CAD build for the part. Positions are in the model's coordinates, mm. Face numbers are marked on the shaded views. A direction names the side the tool comes from. Round coordinates to 2 decimals unless told otherwise and drop trailing zeros. Loops run counter-clockwise (first coordinate to the right, second up) from the corner with the lowest first, then second, coordinate; pieces in that order, holes last.
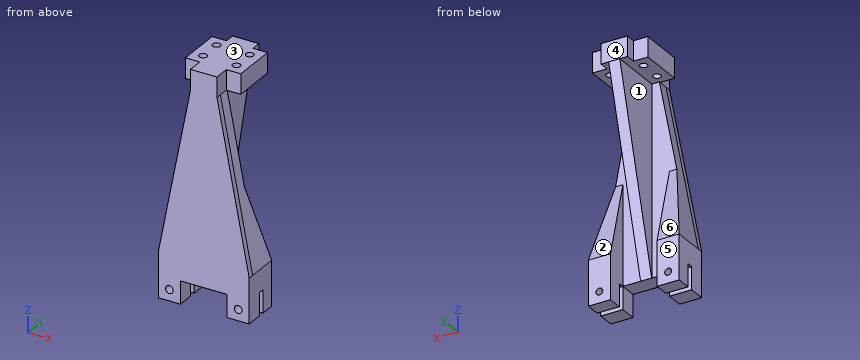
```python
from build123d import *

# Parameters (mm, degrees)
SKETCH1_W            = 41
SKETCH1_H            = 100.5
BOSS_EXTRUDE1_DEPTH  = 5
SKETCH2_W            = 21
SKETCH2_H            = 10.2
CUT_EXTRUDE1_DEPTH   = 109.656569061
SKETCH9_R            = 1.75
CUT_EXTRUDE4_DEPTH   = 109.656569061
CUT_EXTRUDE5_DEPTH   = 109.656569061
BOSS_EXTRUDE4_DEPTH  = 23.9
SKETCH16_W           = 5
SKETCH16_H           = 85.3
BOSS_EXTRUDE5_DEPTH  = 23.9
CUT_EXTRUDE8_DEPTH   = 108.072218619
BOSS_EXTRUDE6_DEPTH  = 28.9
SKETCH25_W           = 6.53486924
SKETCH25_H           = 4.45
CUT_EXTRUDE9_DEPTH   = 108.872424651
SKETCH26_R           = 1.75
CUT_EXTRUDE10_DEPTH  = 113.323016341
SKETCH27_R           = 1.75
BOSS_EXTRUDE7_DEPTH  = 2.5
BOSS_EXTRUDE8_START  = 4
SKETCH28_R           = 1.75
BOSS_EXTRUDE8_DEPTH  = 4
SKETCH29_W           = 10
SKETCH29_H           = 10
BOSS_EXTRUDE9_DEPTH  = 2.7
SKETCH30_W           = 10
SKETCH30_H           = 20.2
BOSS_EXTRUDE10_DEPTH = 6.6
SKETCH31_R           = 1.55
CUT_EXTRUDE11_DEPTH  = 6.6
CHAMFER2_SIZE        = 34.7
CHAMFER2_SIZE_2      = 9.297836977


with BuildPart() as part:
    # Sketch1 → Boss-Extrude1 (new body)
    with BuildSketch(Plane(origin=(0, 0, 0), x_dir=(1, 0, 0), z_dir=(0, 1, 0))):
        with Locations((20.5, 50.25)):
            Rectangle(SKETCH1_W, SKETCH1_H)
    extrude(amount=BOSS_EXTRUDE1_DEPTH)

    # Sketch2 → Cut-Extrude1 (cut, through all)
    with BuildSketch(Plane(origin=(0, 5, 0), x_dir=(1, 0, 0), z_dir=(0, 1, 0))):
        with Locations((20.5, 95.4)):
            Rectangle(SKETCH2_W, SKETCH2_H)
    extrude(amount=-CUT_EXTRUDE1_DEPTH, mode=Mode.SUBTRACT)

    # Sketch9 → Cut-Extrude4 (cut, through all)
    with BuildSketch(Plane(origin=(0, 5, 0), x_dir=(1, 0, 0), z_dir=(0, 1, 0))):
        with Locations(Location((5, 95.5, 0), (0, 0, 270))):
            Circle(SKETCH9_R)
        with Locations(Location((36, 95.5, 0), (0, 0, 270))):
            Circle(SKETCH9_R)
    extrude(amount=-CUT_EXTRUDE4_DEPTH, mode=Mode.SUBTRACT)

    # Sketch11 → Cut-Extrude5 (cut, through all)
    with BuildSketch(Plane(origin=(0, 5, 0), x_dir=(1, 0, 0), z_dir=(0, 1, 0))):
        Polygon((15.5, 0), (0, 80.3), (0, 0), align=None)
        Polygon((25.5, 0), (41, 80.3), (41, 0), align=None)
    extrude(amount=-CUT_EXTRUDE5_DEPTH, mode=Mode.SUBTRACT)

    # Sketch12 → Boss-Extrude4 (add)
    with BuildSketch(Plane(origin=(0, 5, 0), x_dir=(1, 0, 0), z_dir=(0, 1, 0))):
        Polygon((25.5, 0), (15.5, 0), (14.53486924, 5), (26.46513076, 5), align=None)
    extrude(amount=BOSS_EXTRUDE4_DEPTH)

    # Sketch16 → Boss-Extrude5 (add)
    with BuildSketch(Plane(origin=(0, 5, 0), x_dir=(1, 0, 0), z_dir=(0, 1, 0))):
        with Locations((20.5, 47.65)):
            Rectangle(SKETCH16_W, SKETCH16_H)
    extrude(amount=BOSS_EXTRUDE5_DEPTH)

    # Sketch17 → Cut-Extrude8 (cut, through all)
    with BuildSketch(Plane.ZY.offset(-18)):
        Polygon((-90.4, 5), (-5, 28.9), (-90.3, 28.9), align=None)
    extrude(amount=-CUT_EXTRUDE8_DEPTH, mode=Mode.SUBTRACT)

    # Sketch23 → Boss-Extrude6 (add)
    with BuildSketch(Plane(origin=(0, 28.9, 0), x_dir=(1, 0, 0), z_dir=(0, 1, 0))):
        Polygon((26.46513076, 5), (33, 5), (33, 0), (25.5, 0), align=None)
        Polygon((14.53486924, 5), (8, 5), (8, 0), (15.5, 0), align=None)
    extrude(amount=-BOSS_EXTRUDE6_DEPTH)

    # Sketch25 → Cut-Extrude9 (cut, through all)
    with BuildSketch(Plane(origin=(0, 0, -5), x_dir=(-1, 0, 0), z_dir=(0, 0, -1))):
        with Locations((-11.26743462, 2.225)):
            Rectangle(SKETCH25_W, SKETCH25_H)
        with Locations((-29.73256538, 2.225)):
            Rectangle(SKETCH25_W, SKETCH25_H)
        with Locations((-11.26743462, 26.675)):
            Rectangle(SKETCH25_W, SKETCH25_H)
        with Locations((-29.73256538, 26.675)):
            Rectangle(SKETCH25_W, SKETCH25_H)
    extrude(amount=-CUT_EXTRUDE9_DEPTH, mode=Mode.SUBTRACT)

    # Sketch26 → Cut-Extrude10 (cut, through all)
    with BuildSketch(Plane.XY):
        with Locations((13, 19.45)):
            Circle(SKETCH26_R)
        with Locations((28, 19.45)):
            Circle(SKETCH26_R)
        with Locations((13, 9.45)):
            Circle(SKETCH26_R)
        with Locations((28, 9.45)):
            Circle(SKETCH26_R)
    extrude(amount=-CUT_EXTRUDE10_DEPTH, mode=Mode.SUBTRACT)

    # Sketch27 → Boss-Extrude7 (add)
    with BuildSketch(Plane.XZ):
        Polygon((26.46513076, -5), (26.46513076, 0), (14.53486924, 0), (14.53486924, -5), (0, -80.3), (0, -100.5), (10, -100.5), (10, -90.3), (31, -90.3), (31, -100.5), (41, -100.5), (41, -80.3), align=None)
        with Locations(Location((5, -95.5, 0), (0, 0, 90))):
            Circle(SKETCH27_R, mode=Mode.SUBTRACT)
        with Locations(Location((36, -95.5, 0), (0, 0, 90))):
            Circle(SKETCH27_R, mode=Mode.SUBTRACT)
    extrude(amount=BOSS_EXTRUDE7_DEPTH)

    # Sketch28 → Boss-Extrude8 (add)
    with BuildSketch(Plane.XY.offset(BOSS_EXTRUDE8_START)):
        Polygon((26.46513076, -2.5), (26.46513076, 4.45), (33, 4.45), (33, 24.45), (26.46513076, 24.45), (26.46513076, 28.9), (14.53486924, 28.9), (14.53486924, 24.45), (8, 24.45), (8, 4.45), (14.53486924, 4.45), (14.53486924, -2.5), align=None)
        with Locations((28, 9.45)):
            Circle(SKETCH28_R, mode=Mode.SUBTRACT)
        with Locations((13, 9.45)):
            Circle(SKETCH28_R, mode=Mode.SUBTRACT)
        with Locations((28, 19.45)):
            Circle(SKETCH28_R, mode=Mode.SUBTRACT)
        with Locations((13, 19.45)):
            Circle(SKETCH28_R, mode=Mode.SUBTRACT)
    extrude(amount=-BOSS_EXTRUDE8_DEPTH)

    # Sketch29 → Boss-Extrude9 (add)
    with BuildSketch(Plane(origin=(0, 5, 0), x_dir=(1, 0, 0), z_dir=(0, 1, 0))):
        with Locations((36, 85.3)):
            Rectangle(SKETCH29_W, SKETCH29_H)
        with Locations((5, 85.3)):
            Rectangle(SKETCH29_W, SKETCH29_H)
    extrude(amount=BOSS_EXTRUDE9_DEPTH)

    # Sketch30 → Boss-Extrude10 (add)
    with BuildSketch(Plane(origin=(0, 7.7, 0), x_dir=(1, 0, 0), z_dir=(0, 1, 0))):
        with Locations((5, 90.4)):
            Rectangle(SKETCH30_W, SKETCH30_H)
        with Locations((36, 90.4)):
            Rectangle(SKETCH30_W, SKETCH30_H)
    extrude(amount=BOSS_EXTRUDE10_DEPTH)

    # Sketch31 → Cut-Extrude11 (cut)
    with BuildSketch(Plane(origin=(0, 14.3, 0), x_dir=(1, 0, 0), z_dir=(0, 1, 0))):
        with Locations(Location((36, 95.5, 0), (0, 0, 270))):
            Circle(SKETCH31_R)
        with Locations(Location((5, 95.5, 0), (0, 0, 270))):
            Circle(SKETCH31_R)
    extrude(amount=-CUT_EXTRUDE11_DEPTH, mode=Mode.SUBTRACT)

    # Chamfer2
    # the kernel refuses this chamfer: 34.7, 9.297836977 mm, written as the material it adds along each edge
    with BuildSketch(Plane(origin=(41, 5, -80.3), x_dir=(0, -0.009967146577156432, 0.9999503267608395), z_dir=(-1, 0, 0))) as chamfer2_piece_1_section:
        Polygon((CHAMFER2_SIZE * 0.999950326761, CHAMFER2_SIZE * 0.00996714657716), (-CHAMFER2_SIZE_2 * 0.00996714657754, CHAMFER2_SIZE_2 * 0.9999503268), (0, 0), align=None)
    chamfer2_piece_1 = extrude(amount=10, mode=Mode.PRIVATE)
    chamfer2_piece_1 = split(chamfer2_piece_1, bisect_by=Plane(origin=(38.932419972, 8.049756371, -69.588601533), z_dir=(-0.9818753883596208, 0, -0.1895276278900885)), keep=Keep.TOP, mode=Mode.PRIVATE)
    add(chamfer2_piece_1)
    with BuildSketch(Plane(origin=(41, 5, -80.3), x_dir=(0, -0.009967146577156432, 0.9999503267608395), z_dir=(-1, 0, 0))) as chamfer2_piece_2_section:
        Polygon((CHAMFER2_SIZE * 0.999950326761, CHAMFER2_SIZE * 0.00996714657716), (-CHAMFER2_SIZE_2 * 0.00996714657754, CHAMFER2_SIZE_2 * 0.9999503268), (0, 0), align=None)
    chamfer2_piece_2 = extrude(amount=100.106238486, mode=Mode.PRIVATE)
    chamfer2_piece_2 = split(chamfer2_piece_2, bisect_by=Plane(origin=(2.067580028, 8.049756371, -69.588601533), z_dir=(0.9818753883596207, 0, -0.18952762789008884)), keep=Keep.TOP, mode=Mode.PRIVATE)
    chamfer2_piece_2 = split(chamfer2_piece_2, bisect_by=Plane(origin=(0, 8.049756371, -70.340774245), z_dir=(1, 0, 0)), keep=Keep.TOP, mode=Mode.PRIVATE)
    chamfer2_piece_2 = split(chamfer2_piece_2, bisect_by=Plane(origin=(10, 8.049756371, -70.340774245), z_dir=(-1, 0, 0)), keep=Keep.TOP, mode=Mode.PRIVATE)
    add(chamfer2_piece_2)
    with BuildSketch(Plane(origin=(0, 5, -80.3), x_dir=(0, -0.009967146577156432, 0.9999503267608395), z_dir=(1, 0, 0))) as chamfer2_piece_3_section:
        Polygon((CHAMFER2_SIZE * 0.999950326761, -CHAMFER2_SIZE * 0.00996714657716), (-CHAMFER2_SIZE_2 * 0.00996714657754, -CHAMFER2_SIZE_2 * 0.9999503268), (0, 0), align=None)
    chamfer2_piece_3 = extrude(amount=10, mode=Mode.PRIVATE)
    chamfer2_piece_3 = split(chamfer2_piece_3, bisect_by=Plane(origin=(2.067580028, 8.049756371, -69.588601533), z_dir=(0.9818753883596207, 0, -0.18952762789008884)), keep=Keep.TOP, mode=Mode.PRIVATE)
    add(chamfer2_piece_3)
    with BuildSketch(Plane(origin=(0, 5, -80.3), x_dir=(0, -0.009967146577156432, 0.9999503267608395), z_dir=(1, 0, 0))) as chamfer2_piece_4_section:
        Polygon((CHAMFER2_SIZE * 0.999950326761, -CHAMFER2_SIZE * 0.00996714657716), (-CHAMFER2_SIZE_2 * 0.00996714657754, -CHAMFER2_SIZE_2 * 0.9999503268), (0, 0), align=None)
    chamfer2_piece_4 = extrude(amount=100.106238486, mode=Mode.PRIVATE)
    chamfer2_piece_4 = split(chamfer2_piece_4, bisect_by=Plane(origin=(38.932419972, 8.049756371, -69.588601533), z_dir=(-0.9818753883596208, 0, -0.1895276278900885)), keep=Keep.TOP, mode=Mode.PRIVATE)
    chamfer2_piece_4 = split(chamfer2_piece_4, bisect_by=Plane(origin=(31, 8.049756371, -70.340774245), z_dir=(1, 0, 0)), keep=Keep.TOP, mode=Mode.PRIVATE)
    chamfer2_piece_4 = split(chamfer2_piece_4, bisect_by=Plane(origin=(41, 8.049756371, -70.340774245), z_dir=(-1, 0, 0)), keep=Keep.TOP, mode=Mode.PRIVATE)
    add(chamfer2_piece_4)


solid = part.part
```
Item 1: Probe line 1 (Y direction, x = 28, z = -2.5); line 2 (X direction, y = 11.25, z = -95.5); line 3 (Y direction, x = 33.5, z = -96). List the from-to ranges inside material, lowest first.
Answers follow:
line 1: y = 4.45 to 7.7, 11.2 to 17.7, 21.2 to 24.45
line 2: x = 0 to 3.45, 6.55 to 10, 31 to 34.45, 37.55 to 41
line 3: y = -2.5 to 5, 7.7 to 14.3
Item 2: Cut at D-D, the plane z = -33. Give the cut face in (x, y), plus the area to 3 significant figures.
Answers follow:
outline: (9.13, -2.5) - (31.87, -2.5) - (31.87, 5) - (23, 5) - (23, 21.06) - (18, 21.06) - (18, 5) - (9.13, 5) - close
area: 251 mm2
Item 3: 3-axis set-ups, long thin cutter, end or side, ignore diameter. For the marked faces 4, 5 and 6: which of +Z, -Z, +X, -X, +Y, -Y reach the whole face in a straight line?
Answers follow:
face 4: +Z, -Z, +X, -X, +Y
face 5: -Z, +X, -X, +Y
face 6: -X, +Y
Item 4: Cut at B-B, the plane y = 9.45. Give the cut face in (x, z), plus the area to 3 significant figures.
Answers follow:
outline: (0, -100.5) - (10, -100.5) - (10, -62.21) - (3.49, -62.21) - (0, -80.3) - close; (8, -5) - (11.25, -5) - (11.25, 4) - (8, 4) - close; (14.75, -5) - (18, -5) - (18, -74.5) - (23, -74.5) - (23, -5) - (26.25, -5) - (26.25, 4) - (14.75, 4) - close; (29.75, -5) - (33, -5) - (33, 4) - (29.75, 4) - close; (31, -100.5) - (41, -100.5) - (41, -80.3) - (37.51, -62.21) - (31, -62.21) - close; hole circle Ø3.1 at (5, -95.5); hole circle Ø3.1 at (36, -95.5)
area: 1,200 mm2
Item 5: Cut at C-C, the plane y = 16. Give the cut face in (x, z).
Answers follow:
outline: (8, -5) - (18, -5) - (18, -51.09) - (23, -51.09) - (23, -5) - (33, -5) - (33, 4) - (8, 4) - close
Item 6: Cut at A-A, the plane x = 36. State how many separate pieces and enclosed holes the cut face has, plus the area to 3 significant figures.
Answers follow:
separate pieces: 3
enclosed holes: 0
area: 610 mm2
Item 7: Two-plate mould, pull along Z, no slides. Class the marked faces 1, 2 and 3: released by +Z, released by -Z, zero draft, split by the parting line, or undercut.
Answers follow:
face 1: zero draft
face 2: undercut
face 3: released by +Z
Item 8: Flat gauge pins, fed straight in: P1, Ø3, axis at x = 37.5, z = -90, coming from the +Y side; P2, Ø3, axis at y = 24.5, z = -22, coming from the -X side; P3, Ø4.5, axis at x = 28, y = 19.45, coming from the -Z side. Where does each tip first touch, or does it go through?
Answers follow:
P1: stops at y = 14.3
P2: stops at x = 18
P3: stops at z = -5
